Read the model definition and answer for the solid it produces. Units are mm, in the model's axes. A direction names the side the tool comes from. Give positions to 0.01 mm unless a question says otherwise; leave off trailing zeros. Order: outer loops, then holes, each group sorted by start corner. A loop starts at its lowest first (then second) coordinate and runs counter-clockwise, first axis right, second up. Notation, with made-up numbers: (-24, 34.25) - (16, 34.25) arc R36 cw to (16, 73.25) - close; hole circle Ø7 at (-7.5, -39). An arc over 180 degrees is marked (long way). Write each question's results on one line, items separated by ' | '. Start each with the question number.
Q1. Find section C-C on z = 25.25. Give the vertices of the cut face in (x, y).
Q2. A tool of negligible diameter and unlimited length cuts with its end or side. For faces 1 (the face through (-0.938, -4.223, 13.398)), 2 (the face through (-4.76, 0.21, 23.75)), 3 (the face through (-0.702, -3.161, 0.216)), from which of +Z, -Z, +X, -X, +Y, -Y can it reach the whole face along a straight path? Write none if from no direction.
Q3. For a pull along X with two mould halves and no side action, classify faces 4 (the face through (3, -4, 28.575)), 5 (the face through (5.882, 1.852, 25.308)), 6 (the face through (-0.207, 1.574, 9.392)) as +X half, -X half, draft (parallel to the pull), parting line (faces both ways), or undercut.
Q4. Find the intervals of material crossed by line 1 along Y through (x, z) = (0, 25.5); line 2 along Y through (x, z) = (-16.5, 6.5); line 3 along X through (y, z) = (8.5, 7.25), in increasing order. Write a range as from..to.
Q5. Flat-ended cylindrical pins translate along their axes: P1, Ø1.5, axis at y = -5, z = 6, coming from the +X side; P2, Ø1.5, axis at y = 19, z = 7, coming from the +X side; P3, Ø3, axis at x = 16, z = 8, coming from the -Y side. Find the tip coordinate at first contact, or state that the pin passes through.
Q6. Find section A-A on y = 0. Give the vertices of the cut face in (x, z) (3 decimals), and give its area (3 significant figures).
from build123d import *


with BuildPart() as f1:
    # F0 (on Front) → F1 (revolve)
    with BuildSketch(Plane.XZ):
        with BuildLine():
            Line((6.166445, 28.575), (4.762754, 28.575))
            Line((4.762754, 28.575), (4.762754, 19.05))
            Line((4.762754, 19.05), (1.587754, 19.05))
            Line((1.587754, 19.05), (1.587754, 7.416361))
            Line((1.587754, 7.416361), (1.587754, 0))
            Line((1.587754, 0), (27.974581, 3.457336))
            ThreePointArc((27.974581, 3.457336), (30.464123, 3.530209), (31.75, 5.663198))
            Line((31.75, 5.663198), (31.75, 5.886738))
            ThreePointArc((31.75, 5.886738), (28.85973, 8.358248), (26.596049, 5.302472))
            Line((26.596049, 5.302472), (5.082258, 1.326307))
            ThreePointArc((5.082258, 1.326307), (3.203314, 2.517782), (2.43266, 4.604917))
            Line((2.43266, 4.604917), (6.166445, 21.947781))
            Line((6.166445, 21.947781), (6.166445, 28.575))
        make_face()
    revolve(axis=Axis((0, 0, 14.2875), (0, 0, 1)))


solid = f1.part
Working result:
1) outline: circle Ø12.33 at (0, 0); hole circle Ø9.53 at (0, 0)
2) face 1: none | face 2: +Z | face 3: -Z
3) face 4: draft | face 5: parting line | face 6: undercut
4) line 1: -6.17..-4.76, 4.76..6.17 | line 2: -27.01..-20.94, 20.94..27.01 | line 3: -30.12..-25.64, 25.64..30.12
5) P1: x = 31.46 | P2: x = 25.74 | P3: y = -27.71
6) outline: (-31.75, 5.663) arc R2.6 ccw to (-27.975, 3.457) - (-1.588, 0) - (-1.588, 19.05) - (-4.763, 19.05) - (-4.763, 28.575) - (-6.166, 28.575) - (-6.166, 21.948) - (-2.433, 4.605) arc R3.474 cw to (-5.082, 1.326) - (-26.596, 5.302) arc R2.6 ccw (long way) to (-31.75, 5.887) - close; (1.588, 0) - (27.975, 3.457) arc R2.6 ccw to (31.75, 5.663) - (31.75, 5.887) arc R2.6 ccw (long way) to (26.596, 5.302) - (5.082, 1.326) arc R3.474 cw to (2.433, 4.605) - (6.166, 21.948) - (6.166, 28.575) - (4.763, 28.575) - (4.763, 19.05) - (1.588, 19.05) - close | area: 219 mm²
